Read the model definition and answer for the solid it produces. Units are mm, in the model's axes. A direction names the side the tool comes from. Coordinates: 2 decimals unless noted, no trailing zeros. Write each loop counter-clockwise with the first axis right and the second up, starting at its lowest first coordinate (ties: lowest second). Pieces come first, ordered by that corner, then holes.
(1) Which of the six approach directions +Z, -Z, +X, -X, +Y, -Y give full straight-line access (tool end or side, diameter ignored) to faces 4 (the flat face through (0, 0, 2)), 5 (the flat face through (0, 0, 5))?
(2) Find the intervals of material crossed by probe 1 along Y at (x, z) = (-0.1, -3.75); probe 2 along Y at (x, z) = (0, -0.5); probe 3 along X at (y, z) = (0.9, 0.75), in increasing order.
(3) The mould has two halves that part along X. Classify faces 1 (the cylindrical face through (0, -1, -1)), 2 (the flat face through (1, 1, -5)), 3 (the conical face through (-0.45, 2.03, -0.18)): +X half, -X half, draft (parallel to the pull), parting line (faces both ways), or undercut.
(4) Section A-A on x = 0 is taken. Write down the section's boundary in (y, z), then the cut area to 3 significant figures.
(5) Given pin 1 (1.5 mm diameter, centred on x = -0.5, z = 3, fed in from -Y); pin 2 (1 mm diameter, centred on x = -1.5, z = -1, fed in from +Y), each flat-ended and moving along its own axis, determine where each tip first touches the part or whether it passes through.
(6) Section C-C on z = -1.75 is taken. Write down the section's boundary in (x, y), then the cut area to 3 significant figures.
(7) Section D-D on z = 4.75 is taken. Write down the section's boundary in (x, y), then the cut area to 3 significant figures.
Autodesk Inventor part; units mm, degrees
ref_plane "YZ Plane" through (0, 0, 0) normal (1, 0, 0) x (0, 1, 0)
ref_plane "XZ Plane" through (0, 0, 0) normal (0, 1, 0) x (-1, 0, 0)
ref_plane "XY Plane" through (0, 0, 0) normal (0, 0, 1) x (1, 0, 0)
sketch "Sketch1" plane through (0, 0, 0) normal (0, 1, 0) x (-1, 0, 0)
  line L0 (0, 2) -> (0, 5)
  line L1 (0, 5) -> (-1.6251, 5)
  line L2 (-1.6251, 5) -> (-2.5, -5)
  line L3 (-2.5, -5) -> (-1, -5)
  line L4 (-1, -5) -> (-1, 2)
  line L5 (-1, 2) -> (0, 2)
  point P0 (0, 0)
  point P1 (-2.0626, 0)
  dimension "d0" = 10
  dimension "d1" = 2
  dimension "d2" = 7
  dimension "d3" = 5
  dimension "d4" = 5
revolve "Revolution1" add sketch "Sketch1" angle 360 about axis through (0, 0, 2) along (0, 0, 1)
fillet "Fillet1" radius 0.5 1 edges at (-1.6251, 0, 5)
fillet "Fillet2" radius 0.2 1 edges at (-2.5, 0, -5)
properties part number "Locking Pin Lever Rubber" material "Rubber"
Response:
1. face 4: -Z
1. face 5: +Z, +X, -X, +Y, -Y
2. probe 1: y = -2.39 to -0.99, 0.99 to 2.39
2. probe 2: y = -2.11 to -1, 1 to 2.11
2. probe 3: x = -1.78 to -0.44, 0.44 to 1.78
3. face 1: undercut
3. face 2: draft
3. face 3: parting line
4. outline: (-2.48, -4.78) arc R0.2 ccw to (-2.28, -5) - (-1, -5) - (-1, 2) - (1, 2) - (1, -5) - (2.28, -5) arc R0.2 ccw to (2.48, -4.78) - (1.67, 4.54) arc R0.5 ccw to (1.17, 5) - (-1.17, 5) arc R0.5 ccw to (-1.67, 4.54) - close
4. area: 27.1 mm2
5. pin 1: stops at y = -1.85
5. pin 2: stops at y = 1.91
6. outline: circle Ø4.43 at (0, 0); hole circle Ø2 at (0, 0)
6. area: 12.3 mm2
7. outline: circle Ø3.2 at (0, 0)
7. area: 8.04 mm2
